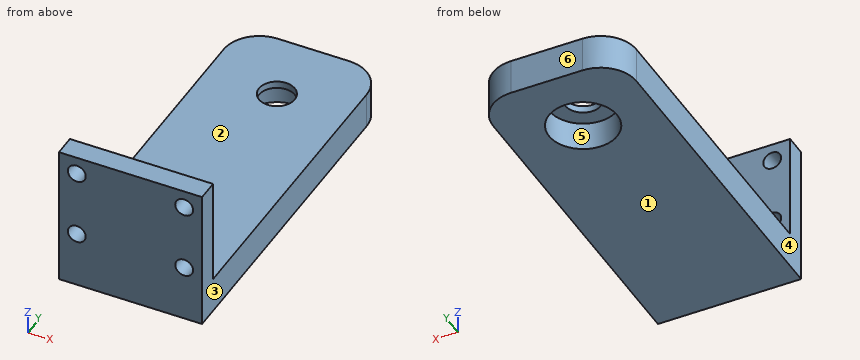
from build123d import *

# Parameters (mm, degrees)
SKETCH_1_W          = 40
SKETCH_1_H          = 30
EXTRUDE_1_DEPTH     = 10
SKETCH_2_W          = 20
SKETCH_2_H          = 5
CUT_EXTRUDE_1_DEPTH = 50
SKETCH_3_W          = 40
SKETCH_3_H          = 8
EXTRUDE_2_DEPTH     = 30
SKETCH_4_W          = 40
SKETCH_4_H          = 2
CUT_EXTRUDE_2_DEPTH = 48.16990566
SKETCH_5_R          = 2.5
CUT_EXTRUDE_3_DEPTH = 15
SKETCH_7_R          = 2.5
CUT_EXTRUDE_4_DEPTH = 15
SKETCH_8_W          = 40
SKETCH_8_H          = 100
EXTRUDE_3_DEPTH     = 10
SKETCH_9_R          = 5
CUT_EXTRUDE_5_DEPTH = 103.29369482
FILLET_1_R          = 10
SKETCH_13_R         = 9.5
CUT_EXTRUDE_8_DEPTH = 99.812954616
SKETCH_14_R         = 9.5
SKETCH_14_R_2       = 5
EXTRUDE_5_DEPTH     = 2


with BuildPart() as part:
    # 草图1 → 凸台-拉伸1 (new body)
    with BuildSketch(Plane.XY):
        Rectangle(SKETCH_1_W, SKETCH_1_H)
    extrude(amount=EXTRUDE_1_DEPTH)

    # 草图2 → 切除-拉伸1 (cut)
    with BuildSketch(Plane.XY.offset(10)):
        with BuildLine():
            ThreePointArc((-20, 12.5), (-19.267766953, 14.267766953), (-17.5, 15))
            Line((-17.5, 15), (-20, 15))
            Line((-20, 15), (-20, 12.5))
        make_face()
        with BuildLine():
            ThreePointArc((5, 5), (3.535533906, 8.535533906), (0, 10))
            Line((0, 10), (0, 0))
            ThreePointArc((0, 0), (3.535533906, 1.464466094), (5, 5))
        make_face()
        with BuildLine():
            Line((0, 0), (0, 10))
            ThreePointArc((0, 10), (-5, 5), (0, 0))
        make_face()
        with BuildLine():
            Line((20, 15), (17.5, 15))
            ThreePointArc((17.5, 15), (19.267766953, 14.267766953), (20, 12.5))
            Line((20, 12.5), (20, 15))
        make_face()
        with Locations((10, -12.5)):
            Rectangle(SKETCH_2_W, SKETCH_2_H)
        with Locations((-10, -12.5)):
            Rectangle(SKETCH_2_W, SKETCH_2_H)
    extrude(amount=-CUT_EXTRUDE_1_DEPTH, mode=Mode.SUBTRACT)

    # 草图3 → 凸台-拉伸2 (add)
    with BuildSketch(Plane.XY.offset(10)):
        with Locations((0, -6)):
            Rectangle(SKETCH_3_W, SKETCH_3_H)
    extrude(amount=EXTRUDE_2_DEPTH)

    # 草图4 → 切除-拉伸2 (cut, through all)
    with BuildSketch(Plane.XY.offset(40)):
        with Locations((0, -9)):
            Rectangle(SKETCH_4_W, SKETCH_4_H)
    extrude(amount=-CUT_EXTRUDE_2_DEPTH, mode=Mode.SUBTRACT)

    # 草图5 → 切除-拉伸3 (cut)
    with BuildSketch(Plane(origin=(0, -2, 0), x_dir=(1, 0, 0), z_dir=(0, 1, 0))):
        with Locations(Location((-15, -35, 0), (0, 0, 270))):
            Circle(SKETCH_5_R)
        with Locations(Location((15, -35, 0), (0, 0, 270))):
            Circle(SKETCH_5_R)
    extrude(amount=-CUT_EXTRUDE_3_DEPTH, mode=Mode.SUBTRACT)

    # 草图7 → 切除-拉伸4 (cut)
    with BuildSketch(Plane(origin=(0, -2, 0), x_dir=(1, 0, 0), z_dir=(0, 1, 0))):
        with Locations(Location((-15, -16, 0), (0, 0, 270))):
            Circle(SKETCH_7_R)
        with Locations(Location((15, -16, 0), (0, 0, 270))):
            Circle(SKETCH_7_R)
    extrude(amount=-CUT_EXTRUDE_4_DEPTH, mode=Mode.SUBTRACT)

    # 草图8 → 凸台-拉伸3 (add)
    with BuildSketch(Plane(origin=(0, 0, 0), x_dir=(-1, 0, 0), z_dir=(0, 0, -1))):
        with Locations((0, 42)):
            Rectangle(SKETCH_8_W, SKETCH_8_H)
    extrude(amount=-EXTRUDE_3_DEPTH)

    # 草图9 → 切除-拉伸5 (cut, through all)
    with BuildSketch(Plane(origin=(0, 0, 0), x_dir=(-1, 0, 0), z_dir=(0, 0, -1))):
        with Locations((0, 72)):
            Circle(SKETCH_9_R)
    extrude(amount=-CUT_EXTRUDE_5_DEPTH, mode=Mode.SUBTRACT)

    # 圆角1
    fillet_1_edges = [part.edges().sort_by_distance(p)[0] for p in [
        (-20, 92, 5),
        (20, 92, 5),
    ]]
    fillet(fillet_1_edges, radius=FILLET_1_R)

    # 草图13 → 切除-拉伸8 (cut, through all)
    with BuildSketch(Plane.XY.offset(10)):
        with Locations((0, 72)):
            Circle(SKETCH_13_R)
    extrude(amount=-CUT_EXTRUDE_8_DEPTH, mode=Mode.SUBTRACT)

    # 草图14 → 凸台-拉伸5 (add)
    with BuildSketch(Plane.XY.offset(10)):
        with Locations((0, 72)):
            Circle(SKETCH_14_R)
        with Locations((0, 72)):
            Circle(SKETCH_14_R_2, mode=Mode.SUBTRACT)
    extrude(amount=-EXTRUDE_5_DEPTH)


solid = part.part
The model under review builds one solid part; all positions refer to its coordinate system, in mm. Face numbers are marked on the shaded views. A direction names the side the tool comes from. Coordinates: 2 decimals unless noted, no trailing zeros. Write each loop counter-clockwise with the first axis right and the second up, starting at its lowest first coordinate (ties: lowest second). Pieces come first, ordered by that corner, then holes. Notation, with made-up numbers: M 24.25,38.25 L 79.25,38.25 A12 cw 79.25,55.25 Z; hole C -40,-37.5 d9. An arc over 180 degrees is marked long. Put each result on its own line as item: value.
1) Add section D-D on x = -16. Give the boundary of the cut face in (y, z), then the cut area to 3 significant figures.
Computed:
outline: M -8,0 L 90,0 L 90,10 L -2,10 L -2,13.71 L -8,13.71 Z; M -8,18.29 L -2,18.29 L -2,32.71 L -8,32.71 Z; M -8,37.29 L -2,37.29 L -2,40 L -8,40 Z
area: 1,110 mm2
2) Clearance check with flat-ended pins moving along their axes: pin 1 Ø6.5 at (x, z) = (15, 35) entering from +Y; pin 2 Ø22 at (x, y) = (0, 72) entering from +Z; pin 3 Ø3 at (x, z) = (-15, 35) entering from +Y. State where each tip first meets the part, or that it passes through.
Computed:
pin 1: stops at y = -2
pin 2: stops at z = 10
pin 3: passes through
3) For the marked faces 1 and 2, list the 3-axis set-ups (+Z, -Z, +X, -X, +Y, -Y) from which the entire face can be reached by the end or side of a thin tool; tool diameter is ignored.
Computed:
face 1: -Z, +X, -X, +Y, -Y
face 2: +Z, +X, -X, +Y
4) Add section A-A on y = 72. Give the boundary of the cut face in (x, z), then the cut area to 3 significant figures.
Computed:
outline: M -20,0 L -9.5,0 L -9.5,8 L -5,8 L -5,10 L -20,10 Z; M 5,8 L 9.5,8 L 9.5,0 L 20,0 L 20,10 L 5,10 Z
area: 228 mm2
5) Wall thickness on probe 1 along X at (y, z) = (-3.6, 35); probe 2 along Y at (x, z) = (0, 9); probe 3 along Z at (x, y) = (-16.5, 20.5): over which ranges is each line inside the solid? List them lowest first. Write a range as [from, to].
Computed:
probe 1: x = [-20, -17.5], [-12.5, 12.5], [17.5, 20]
probe 2: y = [-8, 67], [77, 92]
probe 3: z = [0, 10]
6) Draft analysis for pull direction X (two halves, no side actions). For the marked faces 3, 4, 5 and 6, state which applies: released by +X, released by -X, zero draft, split by the parting line, or undercut.
Computed:
face 3: released by +X
face 4: released by -X
face 5: undercut
face 6: zero draft
7) Add section B-B on z = 16. Give the boundary of the cut face in (x, y).
Computed:
outline: M -20,-8 L -17.5,-8 L -17.5,-2 L -20,-2 Z; M -12.5,-8 L 12.5,-8 L 12.5,-2 L -12.5,-2 Z; M 17.5,-8 L 20,-8 L 20,-2 L 17.5,-2 Z
8) Add section C-C on x = 0. Give the boundary of the cut face in (y, z), then the cut area to 3 significant figures.
Computed:
outline: M -8,0 L 62.5,0 L 62.5,8 L 67,8 L 67,10 L -2,10 L -2,40 L -8,40 Z; M 77,8 L 81.5,8 L 81.5,0 L 92,0 L 92,10 L 77,10 Z
area: 1,010 mm2
